```python
from build123d import *

# Parameters (mm, degrees)
BOSS_EXTRUDE1_DEPTH = 12.6
BOSS_EXTRUDE2_DEPTH = 23.1
BOSS_EXTRUDE3_DEPTH = 3.175
SKETCH1_5_W         = 25.4
SKETCH1_5_H         = 3.175
BOSS_EXTRUDE4_DEPTH = 12.7
FILLET1_R           = 5
FILLET2_R           = 8.175
CUT_EXTRUDE1_DEPTH  = 6.35
CUT_EXTRUDE2_REACH  = 386.06
SKETCH3_R           = 2.275
SKETCH4_W           = 23.1
SKETCH4_H           = 3.8
SKETCH4_W_2         = 3.8
SKETCH4_H_2         = 76.45
EXTRUDE_THIN1_DEPTH = 3.15
SKETCH5_R           = 2.875
BOSS_EXTRUDE5_DEPTH = 6.2
BOSS_EXTRUDE5_TAPER = 2
BOSS_EXTRUDE6_DEPTH = 3.28


with BuildPart() as part:
    # Sketch1 → Boss-Extrude1 (new body)
    with BuildSketch(Plane(origin=(0, 0, 0), x_dir=(0, 0, -1), z_dir=(1, 0, 0))):
        Polygon((175.575, -37.35), (175.575, 0), (-175.575, 0), (-175.575, -55.88), (-88.271480231, -55.88), (-73.904922854, -37.35), (-28.686383268, -37.35), (10.475, -37.35), align=None)
    extrude(amount=-BOSS_EXTRUDE1_DEPTH)

    # Sketch1_3 → Boss-Extrude2 (add)
    with BuildSketch(Plane(origin=(0, 0, 0), x_dir=(0, 0, -1), z_dir=(1, 0, 0))):
        Polygon((175.575, 0), (195.675, 25.925), (195.675, 43.925), (199.075, 43.925), (199.075, -81.275), (195.675, -81.275), (195.675, -61.275), (175.575, -37.35), align=None)
    extrude(amount=-BOSS_EXTRUDE2_DEPTH)

    # Sketch1_4 → Boss-Extrude3 (add)
    with BuildSketch(Plane(origin=(0, 0, 0), x_dir=(0, 0, -1), z_dir=(1, 0, 0))):
        Polygon((0.628519769, -50.05), (10.475, -37.35), (-28.686383268, -37.35), (-24.771480231, -50.05), (-24.771480231, -73.025), (0.628519769, -73.025), align=None)
    extrude(amount=-BOSS_EXTRUDE3_DEPTH)

    # Sketch1_5 → Boss-Extrude4 (add)
    with BuildSketch(Plane(origin=(0, 0, 0), x_dir=(0, 0, -1), z_dir=(1, 0, 0))):
        with Locations((-12.071480231, -74.6125)):
            Rectangle(SKETCH1_5_W, SKETCH1_5_H)
    extrude(amount=-BOSS_EXTRUDE4_DEPTH)

    # Fillet1
    fillet1_edges = [part.edges().sort_by_distance(p)[0] for p in [
        (-3.175, -73.025, 12.071480231),
    ]]
    fillet(fillet1_edges, radius=FILLET1_R)

    # Fillet2
    fillet2_edges = [part.edges().sort_by_distance(p)[0] for p in [
        (-6.3, -55.88, 175.575),
        (-6.3, 0, 175.575),
        (0, -76.2, 12.071480231),
    ]]
    fillet(fillet2_edges, radius=FILLET2_R)

    # Sketch2 → Cut-Extrude1 (cut)
    with BuildSketch(Plane.ZY.offset(12.6)):
        with BuildLine():
            Line((-131.125, -32.5875), (222.402046917, -32.5875))
            ThreePointArc((222.402046917, -32.5875), (223.989546917, -34.175), (222.402046917, -35.7625))
            Line((222.402046917, -35.7625), (-131.125, -35.7625))
            ThreePointArc((-131.125, -35.7625), (-132.7125, -34.175), (-131.125, -32.5875))
        make_face()
    extrude(amount=-CUT_EXTRUDE1_DEPTH, mode=Mode.SUBTRACT)

    # Sketch3 → Cut-Extrude2 (cut, up to next)
    with BuildSketch(Plane(origin=(0, 0, -199.075), x_dir=(-1, 0, 0), z_dir=(0, 0, -1)), mode=Mode.PRIVATE) as cut_extrude2_sk1:
        with Locations((11.55, 33.65)):
            Circle(SKETCH3_R)
    cut_extrude2_tool1 = extrude(cut_extrude2_sk1.sketch, amount=-CUT_EXTRUDE2_REACH, mode=Mode.PRIVATE) & part.part
    # Sketch3 → Cut-Extrude2 (cut, up to next)
    with BuildSketch(Plane(origin=(0, 0, -199.075), x_dir=(-1, 0, 0), z_dir=(0, 0, -1)), mode=Mode.PRIVATE) as cut_extrude2_sk2:
        with BuildLine():
            Line((9.3, -72.325), (9.3, -68.275))
            ThreePointArc((9.3, -68.275), (11.55, -66.025), (13.8, -68.275))
            Line((13.8, -68.275), (13.8, -72.325))
            ThreePointArc((13.8, -72.325), (11.55, -74.575), (9.3, -72.325))
        make_face()
    cut_extrude2_tool2 = extrude(cut_extrude2_sk2.sketch, amount=-CUT_EXTRUDE2_REACH, mode=Mode.PRIVATE) & part.part
    add(cut_extrude2_tool1.solids().sort_by_distance((-11.55, 33.65, -199.075))[0], mode=Mode.SUBTRACT)
    add(cut_extrude2_tool2.solids().sort_by_distance((-11.55, -70.3, -199.075))[0], mode=Mode.SUBTRACT)

    # Sketch4 → Extrude-Thin1 (add)
    with BuildSketch(Plane(origin=(0, 0, -199.075), x_dir=(-1, 0, 0), z_dir=(0, 0, -1))):
        with Locations((11.55, -18.675)):
            Rectangle(SKETCH4_W, SKETCH4_H)
        with Locations((11.55, -18.675)):
            Rectangle(SKETCH4_W_2, SKETCH4_H_2)
    extrude(amount=EXTRUDE_THIN1_DEPTH)

    # Sketch5 → Boss-Extrude5 (add)
    with BuildSketch(Plane(origin=(0, 0, 0), x_dir=(0, 0, -1), z_dir=(1, 0, 0))):
        with Locations((-106.425, -43.625)):
            Circle(SKETCH5_R)
    extrude(amount=BOSS_EXTRUDE5_DEPTH, taper=BOSS_EXTRUDE5_TAPER)

    # Sketch6 → Boss-Extrude6 (add)
    with BuildSketch(Plane(origin=(0, 0, 0), x_dir=(1, 0, 0), z_dir=(0, 1, 0))):
        Polygon((-12.6, 175.575), (-15.6, 175.575), (-12.6, -167.4), align=None)
    extrude(amount=-BOSS_EXTRUDE6_DEPTH)


solid = part.part
```
CAD build for the part. Positions are in the model's coordinates, mm. A direction names the side the tool comes from. Coordinates: 2 decimals unless noted, no trailing zeros. Order: outer loops, then holes, each group sorted by start corner. A loop starts at its lowest first (then second) coordinate and runs counter-clockwise, first axis right, second up. Notation, with made-up numbers: M 58,9.5 L 108,9.5 A18 cw 108,24.5 Z; hole C 87.5,63.5 d1. An arc over 180 degrees is marked long. Write each question's results on one line, items separated by ' | '. Start each with the question number.
Q1. Pull direction Y, two halves, no side cores. Call faces 6 (the cylindrical face through (-6.388, -2.331, 173.117)), 7 (the flat face through (-9, -35.762, 24)), 8 (the flat face through (-11.388, -49.48, -185.766)), 9 (the flat face through (-9, 14, -199.075)): +Y half, -Y half, draft (parallel to the pull), parting line (faces both ways), or undercut.
Q2. Cut at A-A (z = -67). List the corners of the cut face in (x, y).
Q3. Cut at B-B (z = 62). List the corners of the cut face in (x, y).
Q4. Drill centre lines: probe 1 along Y at (x, z) = (-11.55, -196.9) (3 decimals); probe 2 along Z at (x, y) = (-0.5, -66.5) (3 decimals); probe 3 along Z at (x, y) = (-8.5, -12) (3 decimals). Where is each one in solid material? Low to high. Write a range as from..to.
Q5. Which spindle directions (+Z, -Z, +X, -X, +Y, -Y) get a long thin tool onto all of the face, cutting with end or side? Do faces 1 (the flat face through (-6, -55.88, 128)), 2 (the flat face through (-18, -19, -175.575)), 3 (the flat face through (-9, -32.588, 20)), 4 (the flat face through (-9, -71, -195.675)), 5 (the flat face through (-6, -28, 175.575)). Say none if no direction does.
Q6. Flat gauge pins, fed straight in: P1, Ø0.9, axis at x = -13.5, z = -76.5, coming from the -Y side; P2, Ø1, axis at x = -15.5, y = -17.5, coming from the +Z side (3 decimals); P3, Ø3.5, axis at x = -5, z = -201, coming from the +Y side (3 decimals). Where does each tip first touch, or does it go through?
Found:
1) face 6: +Y half | face 7: undercut | face 8: -Y half | face 9: draft
2) outline: M -14.65,-3.28 L -12.6,-3.28 L -12.6,-32.59 L -6.25,-32.59 L -6.25,-35.76 L -12.6,-35.76 L -12.6,-37.35 L 0,-37.35 L 0,0 L -14.65,0 Z
3) outline: M -13.52,-3.28 L -12.6,-3.28 L -12.6,-32.59 L -6.25,-32.59 L -6.25,-35.76 L -12.6,-35.76 L -12.6,-37.35 L 0,-37.35 L 0,0 L -13.52,0 Z
4) probe 1: -81.275..-74.575, -66.025..31.375, 35.925..43.925 | probe 2: -199.075..-195.675, -0.629..24.771 | probe 3: -199.075..175.575
5) face 1: +Z, +X, -X, -Y | face 2: +Z, -X, -Y | face 3: +Z, -X | face 4: +X, -X, -Y | face 5: +Z, +X, -X, +Y, -Y
6) P1: y = -3.28 | P2: z = -175.575 | P3: y = -16.775
